from build123d import *

# Parameters (mm, degrees)
SKETCH2_W            = 50.8
SKETCH2_H            = 25.4
SKETCH2_W_2          = 44.45
SKETCH2_H_2          = 19.05
EXTRUDE_THIN1_DEPTH  = 355.6
SKETCH25_W           = 50.8
SKETCH25_H           = 25.4
SKETCH25_W_2         = 44.45
SKETCH25_H_2         = 19.05
BOSS_EXTRUDE14_DEPTH = 25.4
CUT_EXTRUDE9_START   = -25.4
SKETCH28_R           = 6
CUT_EXTRUDE9_DEPTH   = 25.4
SKETCH30_W           = 50.8
SKETCH30_H           = 25.4
CUT_EXTRUDE11_DEPTH  = 38.1


with BuildPart() as part:
    # Sketch2 → Extrude-Thin1 (new body)
    with BuildSketch(Plane(origin=(0, 0, 0), x_dir=(1, 0, 0), z_dir=(0, 1, 0))):
        with Locations((10.213756614, 0.671957672)):
            Rectangle(SKETCH2_W, SKETCH2_H)
        with Locations((10.213756614, 0.671957672)):
            Rectangle(SKETCH2_W_2, SKETCH2_H_2, mode=Mode.SUBTRACT)
    extrude(amount=EXTRUDE_THIN1_DEPTH)

    # Sketch25 → Boss-Extrude14 (add)
    with BuildSketch(Plane.XZ):
        with Locations((10.213756614, -0.671957672)):
            Rectangle(SKETCH25_W, SKETCH25_H)
        with Locations((10.213756614, -0.671957672)):
            Rectangle(SKETCH25_W_2, SKETCH25_H_2, mode=Mode.SUBTRACT)
    extrude(amount=BOSS_EXTRUDE14_DEPTH)

    # Sketch28 → Cut-Extrude9 (cut)
    with BuildSketch(Plane(origin=(0, 0, -13.371957672), x_dir=(-1, 0, 0), z_dir=(0, 0, -1)).offset(CUT_EXTRUDE9_START)):
        with Locations((-10.213756614, 0)):
            Circle(SKETCH28_R)
    extrude(amount=CUT_EXTRUDE9_DEPTH, mode=Mode.SUBTRACT)

    # Sketch30 → Cut-Extrude11 (cut)
    with BuildSketch(Plane(origin=(0, 355.6, 0), x_dir=(1, 0, 0), z_dir=(0, 1, 0))):
        with Locations((10.213756614, 0.671957672)):
            Rectangle(SKETCH30_W, SKETCH30_H)
    extrude(amount=-CUT_EXTRUDE11_DEPTH, mode=Mode.SUBTRACT)


solid = part.part
CAD build for the part. Positions are in the model's coordinates, mm. A direction names the side the tool comes from. Give positions to 0.01 mm unless a question says otherwise; leave off trailing zeros. Write each loop counter-clockwise with the first axis right and the second up, starting at its lowest first coordinate (ties: lowest second). Pieces come first, ordered by that corner, then holes. Notation, with made-up numbers: M -32.75,32.25 L -10.75,32.25 A16 cw -10.75,53.25 Z; hole C 12.25,27 d8. An arc over 180 degrees is marked long. Put each result on its own line as item: value. Start each with the question number.
(1) Band-saw the part on A-A, the plane x = -1.5. Write the cut outline in (y, z).
(2) Band-saw the part on D-D, the plane y = 0. Write the cut outline in (x, z), and give its area (3 significant figures).
(3) Mould opens along Y. For faces 3 (the face through (10, 317.5, -11)), 4 (the face through (4.49, 1.8, -11.76)), 5 (the face through (10, 148, -13.372)) say: +Y half, -Y half, draft (parallel to the pull), parting line (faces both ways), or undercut.
(4) Band-saw the part on C-C, the plane z = 3.25. Write the cut outline in (x, y), and give its area (3 significant figures).
(5) Flat gauge pin, fed straight in: pin 1 Ø6 at (x, z) = (7, -8.5) entering from -Y. Where does the tip first touch, or does it go through?
(6) Which spindle directions (+Z, -Z, +X, -X, +Y, -Y) get a long thin tool onto all of the face, cutting with end or side? Do faces 1 (the face through (10, -25.4, 10)), 2 (the face through (10, 148, 8.853)). Say none if no direction does.
(7) Band-saw the part on B-B, the plane y = 145. Write the cut outline in (x, z).
(8) Probe L1, parallel to Z at x = -8.5, y = 197.5; L2, parallel to X at y = 0, z = -11.55; L3, parallel to X at y = 122.5, z = -9.5. List the from-to ranges inside material, lowest first.
Response values:
1. outline: M -25.4,-13.37 L 317.5,-13.37 L 317.5,-10.2 L -25.4,-10.2 Z; M -25.4,8.85 L 317.5,8.85 L 317.5,12.03 L -25.4,12.03 Z
2. outline: M -15.19,-13.37 L 4.21,-13.37 L 4.21,-10.2 L -12.01,-10.2 L -12.01,8.85 L 4.21,8.85 L 4.21,12.03 L -15.19,12.03 Z; M 16.21,-13.37 L 35.61,-13.37 L 35.61,12.03 L 16.21,12.03 L 16.21,8.85 L 32.44,8.85 L 32.44,-10.2 L 16.21,-10.2 Z
2. area: 367 mm2
3. face 3: +Y half
3. face 4: undercut
3. face 5: draft
4. outline: M -15.19,-25.4 L -12.01,-25.4 L -12.01,317.5 L -15.19,317.5 Z; M 32.44,-25.4 L 35.61,-25.4 L 35.61,317.5 L 32.44,317.5 Z
4. area: 2,180 mm2
5. pin 1: stops at y = -25.4
6. face 1: +Z, -Z, +X, -X, -Y
6. face 2: +Y, -Y
7. outline: M -15.19,-13.37 L 35.61,-13.37 L 35.61,12.03 L -15.19,12.03 Z; hole M -12.01,-10.2 L 32.44,-10.2 L 32.44,8.85 L -12.01,8.85 Z
8. L1: z = -13.37 to -10.2, 8.85 to 12.03
8. L2: x = -15.19 to 4.21, 16.21 to 35.61
8. L3: x = -15.19 to -12.01, 32.44 to 35.61
